For this review, take the finished solid that the model builds, in its own axes (mm). Face numbers are marked on the shaded views. A direction names the side the tool comes from. Give positions to 0.01 mm unless a question says otherwise; leave off trailing zeros. Write each loop counter-clockwise with the first axis right and the second up, starting at its lowest first coordinate (ties: lowest second). Pieces come first, ordered by that corner, then holes.
1) Wall thickness on line 1 along Y through (x, z) = (55, 15.25); line 2 along Y through (x, z) = (58, 17); line 3 along Y through (x, z) = (70, 15.75): over which ranges is each line inside the solid? List them lowest first.
2) For P1, Ø10, axis at y = 32.5, z = 22.5, coming from the +X side; P2, Ø3.5, axis at x = 39, y = 63, coming from the +Z side; P3, Ø9, axis at x = 85, y = 65, coming from the +Z side; P4, Ø2, axis at x = 31.5, z = 20.5, coming from the +Y side, all flat-tipped, find the tip position at first contact; note any pin that passes through.
3) We need section B-B on x = 100. Give the boundary of the cut face in (y, z).
4) We need section C-C on z = 18.75. Give the number of separate pieces and of enclosed holes in the cut face, and give its area (3 significant figures).
5) Machinability: for the marked faces 4, 5 and 6, which of the approach directions +Z, -Z, +X, -X, +Y, -Y give a long, thin tool a straight path to every point of the face, cutting with its end or side? Answer none if there is none.
6) We need section D-D on x = 127.5. Give the boundary of the cut face in (y, z).
7) Draft analysis for pull direction X (two halves, no side actions). For the marked faces 1, 2 and 3, state which applies: pulls with the +X half, pulls with the -X half, needs draft (parallel to the pull), parting line crosses it, or undercut.
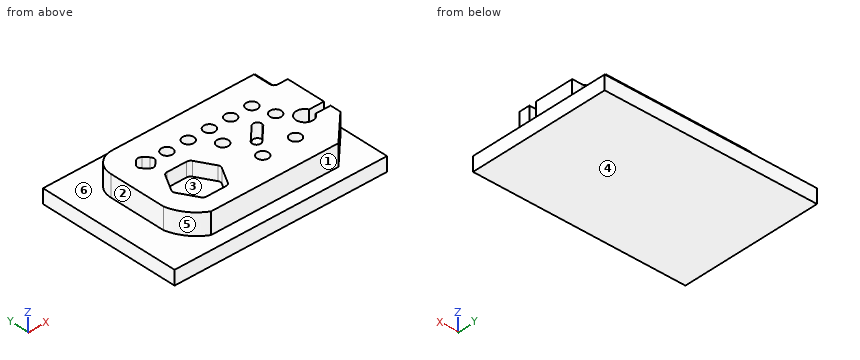
from build123d import *

# Parameters (mm, degrees)
F1_W      = 150
F1_H      = 100
F2_DEPTH  = 10
F3_W      = 125
F3_H      = 75
F4_DEPTH  = 15
F5_R      = 15
F6_SIZE   = 20
F7_W      = 10
F7_H      = 15
F8_DEPTH  = 15
F10_DEPTH = 15
F11_R     = 4
F12_DEPTH = 15
F14_DEPTH = 15
F16_DEPTH = 15
F18_DEPTH = 10
F20_DEPTH = 10
F21_R     = 3
F22_R     = 3


with BuildPart() as f2:
    # F1 (on offset) → F2 (new body)
    with BuildSketch(Plane.XY):
        with Locations((75, 50)):
            Rectangle(F1_W, F1_H)
    extrude(amount=F2_DEPTH)

    # F3 (on face) → F4 (join)
    with BuildSketch(Plane.XY.offset(10)):
        with Locations((82.5, 47.5)):
            Rectangle(F3_W, F3_H)
    extrude(amount=F4_DEPTH)

    # F5
    f5_edges = [f2.edges().sort_by_distance(p)[0] for p in [
        (20, 85, 17.5),
    ]]
    fillet(f5_edges, radius=F5_R)

    # F6
    f6_edges = [f2.edges().sort_by_distance(p)[0] for p in [
        (145, 10, 17.5),
    ]]
    chamfer(f6_edges, length=F6_SIZE)

    # F7 (on face) → F8 (cut)
    with BuildSketch(Plane.XY.offset(25)):
        with Locations((140, 77.5)):
            Rectangle(F7_W, F7_H)
    extrude(amount=-F8_DEPTH, mode=Mode.SUBTRACT)

    # F9 (on face) → F10 (cut, through all)
    with BuildSketch(Plane.XY.offset(25)):
        with BuildLine():
            ThreePointArc((35, 10), (25.3174242293, 18.363068172), (20, 30))
            Line((20, 30), (20, 10))
            Line((20, 10), (35, 10))
        make_face()
    extrude(amount=-F10_DEPTH, mode=Mode.SUBTRACT)

    # F11 (on face) → F12 (cut)
    with BuildSketch(Plane.XY.offset(25)):
        with Locations((55, 65)):
            Circle(F11_R)
        with Locations((70, 65)):
            Circle(F11_R)
        with Locations((85, 65)):
            Circle(F11_R)
        with Locations((100, 65)):
            Circle(F11_R)
        with Locations((115, 65)):
            Circle(F11_R)
        with Locations((119.2491547178, 51.4941885379)):
            Circle(F11_R)
        with Locations((112.352680654, 29.0136292458)):
            Circle(F11_R)
        with Locations((88.8412705623, 28.6256909792)):
            Circle(F11_R)
        with Locations((81.206894066, 50.8664912371)):
            Circle(F11_R)
    extrude(amount=-F12_DEPTH, mode=Mode.SUBTRACT)

    # F13 (on face) → F14 (cut)
    with BuildSketch(Plane.XY.offset(25)):
        Polygon((40, 72.0710678119), (32.9289321881, 65), (40, 57.9289321881), (47.0710678119, 65), align=None)
    extrude(amount=-F14_DEPTH, mode=Mode.SUBTRACT)

    # F15 (on face) → F16 (cut)
    with BuildSketch(Plane.XY.offset(25)):
        with BuildLine():
            Line((134.4543560573, 37.5), (145, 37.5))
            Line((145, 37.5), (145, 42.5))
            Line((145, 42.5), (134.4543560573, 42.5))
            ThreePointArc((134.4543560573, 42.5), (134.8620020617, 41.2794263668), (135, 40))
            ThreePointArc((135, 40), (134.8620020617, 38.7205736332), (134.4543560573, 37.5))
        make_face()
        with BuildLine():
            ThreePointArc((134.4543560573, 42.5), (123, 40), (134.4543560573, 37.5))
            Line((134.4543560573, 37.5), (129, 37.5))
            Line((129, 37.5), (129, 42.5))
            Line((129, 42.5), (134.4543560573, 42.5))
        make_face()
        with BuildLine():
            Line((129, 37.5), (134.4543560573, 37.5))
            ThreePointArc((134.4543560573, 37.5), (134.8620020617, 38.7205736332), (135, 40))
            ThreePointArc((135, 40), (134.8620020617, 41.2794263668), (134.4543560573, 42.5))
            Line((134.4543560573, 42.5), (129, 42.5))
            Line((129, 42.5), (129, 37.5))
        make_face()
    extrude(amount=-F16_DEPTH, mode=Mode.SUBTRACT)

    # F17 (on face) → F18 (cut)
    with BuildSketch(Plane.XY.offset(25)):
        with BuildLine():
            Line((102.8786796564, 52.1213203436), (92.8786796564, 42.1213203436))
            ThreePointArc((92.8786796564, 42.1213203436), (96.1480502971, 42.7716385975), (98, 40))
            ThreePointArc((98, 40), (97.7716385975, 38.8519497029), (97.1213203436, 37.8786796564))
            Line((97.1213203436, 37.8786796564), (107.1213203436, 47.8786796564))
            ThreePointArc((107.1213203436, 47.8786796564), (102.8786796564, 47.8786796564), (102.8786796564, 52.1213203436))
        make_face()
        with BuildLine():
            ThreePointArc((98, 40), (96.1480502971, 42.7716385975), (92.8786796564, 42.1213203436))
            ThreePointArc((92.8786796564, 42.1213203436), (92.8786796564, 37.8786796564), (97.1213203436, 37.8786796564))
            ThreePointArc((97.1213203436, 37.8786796564), (97.7716385975, 38.8519497029), (98, 40))
        make_face()
        with BuildLine():
            ThreePointArc((108, 50), (106.1480502971, 52.7716385975), (102.8786796564, 52.1213203436))
            ThreePointArc((102.8786796564, 52.1213203436), (102.8786796564, 47.8786796564), (107.1213203436, 47.8786796564))
            ThreePointArc((107.1213203436, 47.8786796564), (107.7716385975, 48.8519497029), (108, 50))
        make_face()
    extrude(amount=-F18_DEPTH, mode=Mode.SUBTRACT)

    # F19 (on face) → F20 (cut)
    with BuildSketch(Plane.XY.offset(25)):
        Polygon((40.6571701914, 51.363068172), (31.9969161536, 36.363068172), (40.6571701914, 21.363068172), (57.9776782671, 21.363068172), (66.637932305, 36.363068172), (57.9776782671, 51.363068172), align=None)
    extrude(amount=-F20_DEPTH, mode=Mode.SUBTRACT)

    # F21
    f21_edges = [f2.edges().sort_by_distance(p)[0] for p in [
        (32.928932, 65, 17.5),
        (40, 72.071068, 17.5),
        (47.071068, 65, 17.5),
        (40, 57.928932, 17.5),
        (57.977678, 51.363068, 20),
        (40.65717, 51.363068, 20),
        (31.996916, 36.363068, 20),
        (40.65717, 21.363068, 20),
        (57.977678, 21.363068, 20),
        (66.637932, 36.363068, 20),
    ]]
    fillet(f21_edges, radius=F21_R)

    # F22
    f22_edges = [f2.edges().sort_by_distance(p)[0] for p in [
        (135, 70, 17.5),
    ]]
    fillet(f22_edges, radius=F22_R)


solid = f2.part
Results list:
1. line 1: y = 10 to 21.36, 51.36 to 61, 69 to 85
1. line 2: y = 10 to 21.93, 50.8 to 62.35, 67.65 to 85
1. line 3: y = 10 to 61, 69 to 85
2. P1: stops at x = 145
2. P2: stops at z = 10
2. P3: stops at z = 25
2. P4: stops at y = 84.79
3. outline: (0, 0) - (100, 0) - (100, 10) - (85, 10) - (85, 25) - (69, 25) - (69, 10) - (61, 10) - (61, 25) - (49.24, 25) - (49.24, 15) - (40.76, 15) - (40.76, 25) - (10, 25) - (10, 10) - (0, 10) - close
4. separate pieces: 1
4. enclosed holes: 12
4. area: 7,280 mm2
5. face 4: -Z, +X, -X, +Y, -Y
5. face 5: +Z, -X, -Y
5. face 6: +Z
6. outline: (0, 0) - (100, 0) - (100, 10) - (85, 10) - (85, 25) - (45.81, 25) - (45.81, 10) - (34.19, 10) - (34.19, 25) - (12.5, 25) - (12.5, 10) - (0, 10) - close
7. face 1: needs draft
7. face 2: pulls with the -X half
7. face 3: undercut
